Check sheet for the modelled part. Datum: model origin and axes. Units: mm. Face numbers are marked on the shaded views. A direction names the side the tool comes from. Coordinates: 2 decimals unless noted, no trailing zeros. Loops run counter-clockwise (first coordinate to the right, second up) from the corner with the lowest first, then second, coordinate; pieces in that order, holes last. Notation, with made-up numbers: (-26, 33) -> (-9, 33) arc R15 cw to (-9, 61) -> close; hole circle Ø10 at (19, 20.25). An arc over 180 degrees is marked (long way). Use CSV: the item, a comma, the result in double quotes. Start each with the question number.
1. Sectioned sample at D-D, the plane z = -16. Count the separate pieces of the cut face and the enclosed holes in it, and give its area (3 significant figures).
2. Sectioned sample at C-C, the plane y = -31. Record the cut outline in (x, z), and give its area (3 significant figures).
3. Thickness scan on L1, parallel to X at y = -71.1, z = -20; L2, parallel to X at y = -7.5, z = 33; L3, parallel to Y at x = -12.5, z = -45. Record the ranges inside material, lowest first.
4. Release check for a two-part mould opening along X. For the marked faces 3, 4 and 5 record: pulls with the +X half, pulls with the -X half, needs draft (parallel to the pull), parting line crosses it, or undercut.
5. Sectioned sample at A-A, the plane y = -4.5. Record the cut outline in (x, z), and give its area (3 significant figures).
6. Sectioned sample at B-B, the plane y = -54. Record the cut outline in (x, z).
7. Gauge pin test, flat ends, axial feed: pin 1 (1.8 mm diameter, centred on x = 25.81, z = -25.81, fed in from -Y); pin 2 (5 mm diameter, centred on x = 25.81, z = 25.81, fed in from +Y); pin 3 (8 mm diameter, centred on x = 10, z = 4.5, fed in from +Y). Record the tip position at first contact, or that the pin passes through.
8. Set-up check for the marked faces 1 and 2: record each of +Z, -Z, +X, -X, +Y, -Y from which the full face is reachable in a straight line by a thin tool's end or side.
```python
from build123d import *

# Parameters (mm, degrees)
SKETCH_1_W           = 90
SKETCH_1_H           = 80
SKETCH_1_R           = 30
EXTRUDE_1_DEPTH      = 4
SKETCH_2_R           = 1.5
CUT_EXTRUDE_1_DEPTH  = 4
SKETCH_3_W           = 80
SKETCH_3_H           = 80
EXTRUDE_2_DEPTH      = 4
SKETCH_4_W           = 80
SKETCH_4_H           = 80
EXTRUDE_3_DEPTH      = 4
SKETCH_5_R           = 1.5
CUT_EXTRUDE_2_DEPTH  = 4
SKETCH_6_R           = 20.5
CUT_EXTRUDE_3_DEPTH  = 4
SKETCH_8_W           = 98
SKETCH_8_H           = 80
EXTRUDE_4_DEPTH      = 4
SKETCH_9_R           = 8
CUT_EXTRUDE_5_DEPTH  = 4
SKETCH_10_R          = 2.75
CUT_EXTRUDE_6_DEPTH  = 2
SKETCH_11_W          = 106.087882822
SKETCH_11_H          = 86.695474134
CUT_EXTRUDE_7_DEPTH  = 2
SKETCH_12_W          = 90
SKETCH_12_H          = 80
EXTRUDE_5_DEPTH      = 2
SKETCH_13_W          = 115.80209227
SKETCH_13_H          = 95.07614962
CUT_EXTRUDE_8_DEPTH  = 0.5
SKETCH_14_R          = 12.5
CUT_EXTRUDE_9_DEPTH  = 4
FILLET_1_R           = 2
CUT_EXTRUDE_10_REACH = 131.151
SKETCH_15_R          = 10
SKETCH_16_W          = 90
SKETCH_16_H          = 70
EXTRUDE_6_DEPTH      = 10
SKETCH_17_W          = 90
SKETCH_17_H          = 70
EXTRUDE_7_DEPTH      = 10
SKETCH_19_R          = 2
CUT_EXTRUDE_12_DEPTH = 105.43778052
SKETCH_20_R          = 8
SKETCH_20_R_2        = 7.5
EXTRUDE_8_DEPTH      = 4


with BuildPart() as part:
    # 草图1 → 凸台-拉伸1 (new body)
    with BuildSketch(Plane(origin=(0, 0, 0), x_dir=(1, 0, 0), z_dir=(0, 1, 0))):
        Rectangle(SKETCH_1_W, SKETCH_1_H)
        with Locations(Location((0, 0, 0), (0, 0, 270))):
            Circle(SKETCH_1_R, mode=Mode.SUBTRACT)
    extrude(amount=EXTRUDE_1_DEPTH)

    # 草图2 → 切除-拉伸1 (cut)
    with BuildSketch(Plane(origin=(0, 4, 0), x_dir=(1, 0, 0), z_dir=(0, 1, 0))):
        with Locations(Location((0, 36.5, 0), (0, 0, 270))):
            Circle(SKETCH_2_R)
        with Locations(Location((25.809397513, 25.809397513, 0), (0, 0, 270))):
            Circle(SKETCH_2_R)
        with Locations(Location((36.5, 0, 0), (0, 0, 270))):
            Circle(SKETCH_2_R)
        with Locations(Location((25.809397513, -25.809397513, 0), (0, 0, 270))):
            Circle(SKETCH_2_R)
        with Locations(Location((0, -36.5, 0), (0, 0, 270))):
            Circle(SKETCH_2_R)
        with Locations(Location((-25.809397513, -25.809397513, 0), (0, 0, 270))):
            Circle(SKETCH_2_R)
        with Locations(Location((-36.5, 0, 0), (0, 0, 270))):
            Circle(SKETCH_2_R)
        with Locations(Location((-25.809397513, 25.809397513, 0), (0, 0, 270))):
            Circle(SKETCH_2_R)
    extrude(amount=-CUT_EXTRUDE_1_DEPTH, mode=Mode.SUBTRACT)

    # 草图3 → 凸台-拉伸2 (add)
    with BuildSketch(Plane(origin=(45, 0, 0), x_dir=(0, 0, -1), z_dir=(1, 0, 0))):
        with Locations((0, -36)):
            Rectangle(SKETCH_3_W, SKETCH_3_H)
    extrude(amount=EXTRUDE_2_DEPTH)

    # 草图4 → 凸台-拉伸3 (add)
    with BuildSketch(Plane.ZY.offset(45)):
        with Locations((0, -36)):
            Rectangle(SKETCH_4_W, SKETCH_4_H)
    extrude(amount=EXTRUDE_3_DEPTH)

    # 草图5 → 切除-拉伸2 (cut)
    with BuildSketch(Plane(origin=(49, 0, 0), x_dir=(0, 0, -1), z_dir=(1, 0, 0))):
        with Locations((-24, -36)):
            Circle(SKETCH_5_R)
        with Locations((-12, -15.215390309)):
            Circle(SKETCH_5_R)
        with Locations((12, -15.215390309)):
            Circle(SKETCH_5_R)
        with Locations((24, -36)):
            Circle(SKETCH_5_R)
        with Locations((12, -56.784609691)):
            Circle(SKETCH_5_R)
        with Locations((-12, -56.784609691)):
            Circle(SKETCH_5_R)
    extrude(amount=-CUT_EXTRUDE_2_DEPTH, mode=Mode.SUBTRACT)

    # 草图6 → 切除-拉伸3 (cut)
    with BuildSketch(Plane(origin=(49, 0, 0), x_dir=(0, 0, -1), z_dir=(1, 0, 0))):
        with Locations((0, -36)):
            Circle(SKETCH_6_R)
    extrude(amount=-CUT_EXTRUDE_3_DEPTH, mode=Mode.SUBTRACT)

    # 草图8 → 凸台-拉伸4 (add)
    with BuildSketch(Plane.XZ.offset(76)):
        Rectangle(SKETCH_8_W, SKETCH_8_H)
    extrude(amount=-EXTRUDE_4_DEPTH)

    # 草图9 → 切除-拉伸5 (cut)
    with BuildSketch(Plane.ZY.offset(49)):
        with Locations((0, -36)):
            Circle(SKETCH_9_R)
    extrude(amount=-CUT_EXTRUDE_5_DEPTH, mode=Mode.SUBTRACT)

    # 草图10 → 切除-拉伸6 (cut)
    with BuildSketch(Plane(origin=(0, 4, 0), x_dir=(1, 0, 0), z_dir=(0, 1, 0))):
        with Locations(Location((-25.809397513, 25.809397513, 0), (0, 0, 270))):
            Circle(SKETCH_10_R)
        with Locations(Location((0, 36.5, 0), (0, 0, 270))):
            Circle(SKETCH_10_R)
        with Locations(Location((25.809397513, 25.809397513, 0), (0, 0, 270))):
            Circle(SKETCH_10_R)
        with Locations(Location((36.5, 0, 0), (0, 0, 270))):
            Circle(SKETCH_10_R)
        with Locations(Location((25.809397513, -25.809397513, 0), (0, 0, 270))):
            Circle(SKETCH_10_R)
        with Locations(Location((0, -36.5, 0), (0, 0, 270))):
            Circle(SKETCH_10_R)
        with Locations(Location((-25.809397513, -25.809397513, 0), (0, 0, 270))):
            Circle(SKETCH_10_R)
        with Locations(Location((-36.5, 0, 0), (0, 0, 270))):
            Circle(SKETCH_10_R)
    extrude(amount=-CUT_EXTRUDE_6_DEPTH, mode=Mode.SUBTRACT)

    # 草图11 → 切除-拉伸7 (cut)
    with BuildSketch(Plane.XZ.offset(76)):
        with Locations((0.826302958, 0.912583938)):
            Rectangle(SKETCH_11_W, SKETCH_11_H)
    extrude(amount=-CUT_EXTRUDE_7_DEPTH, mode=Mode.SUBTRACT)

    # 草图12 → 凸台-拉伸5 (add)
    with BuildSketch(Plane(origin=(0, -72, 0), x_dir=(1, 0, 0), z_dir=(0, 1, 0))):
        Rectangle(SKETCH_12_W, SKETCH_12_H)
    extrude(amount=EXTRUDE_5_DEPTH)

    # 草图13 → 切除-拉伸8 (cut)
    with BuildSketch(Plane(origin=(0, 4, 0), x_dir=(1, 0, 0), z_dir=(0, 1, 0))):
        with Locations((-2.14666103, 3.125340558)):
            Rectangle(SKETCH_13_W, SKETCH_13_H)
    extrude(amount=-CUT_EXTRUDE_8_DEPTH, mode=Mode.SUBTRACT)

    # 草图14 → 切除-拉伸9 (cut)
    with BuildSketch(Plane.XZ.offset(74)):
        with Locations(Location((-29, 20, 0), (0, 0, 270))):
            Circle(SKETCH_14_R)
        with Locations(Location((29, 20, 0), (0, 0, 270))):
            Circle(SKETCH_14_R)
        with Locations(Location((0, 0, 0), (0, 0, 270))):
            Circle(SKETCH_14_R)
        with Locations(Location((-29, -20, 0), (0, 0, 270))):
            Circle(SKETCH_14_R)
        with Locations(Location((29, -20, 0), (0, 0, 270))):
            Circle(SKETCH_14_R)
    extrude(amount=-CUT_EXTRUDE_9_DEPTH, mode=Mode.SUBTRACT)

    # 圆角1
    fillet_1_edges = [part.edges().sort_by_distance(p)[0] for p in [
        (-49, -74, 0),
        (49, -74, 0),
        (49, 3.5, 0),
        (-49, 3.5, 0),
    ]]
    fillet(fillet_1_edges, radius=FILLET_1_R)

    # 草图15 → 切除-拉伸10 (cut, up to next)
    with BuildSketch(Plane.ZY.offset(49), mode=Mode.PRIVATE) as cut_extrude_10_sk1:
        with Locations((-20, -16.5)):
            Circle(SKETCH_15_R)
    cut_extrude_10_tool1 = extrude(cut_extrude_10_sk1.sketch, amount=-CUT_EXTRUDE_10_REACH, mode=Mode.PRIVATE) & part.part
    # 草图15 → 切除-拉伸10 (cut, up to next)
    with BuildSketch(Plane.ZY.offset(49), mode=Mode.PRIVATE) as cut_extrude_10_sk2:
        with Locations((20, -16.5)):
            Circle(SKETCH_15_R)
    cut_extrude_10_tool2 = extrude(cut_extrude_10_sk2.sketch, amount=-CUT_EXTRUDE_10_REACH, mode=Mode.PRIVATE) & part.part
    # 草图15 → 切除-拉伸10 (cut, up to next)
    with BuildSketch(Plane.ZY.offset(49), mode=Mode.PRIVATE) as cut_extrude_10_sk3:
        with Locations((20, -54)):
            Circle(SKETCH_15_R)
    cut_extrude_10_tool3 = extrude(cut_extrude_10_sk3.sketch, amount=-CUT_EXTRUDE_10_REACH, mode=Mode.PRIVATE) & part.part
    # 草图15 → 切除-拉伸10 (cut, up to next)
    with BuildSketch(Plane.ZY.offset(49), mode=Mode.PRIVATE) as cut_extrude_10_sk4:
        with Locations((-20, -54)):
            Circle(SKETCH_15_R)
    cut_extrude_10_tool4 = extrude(cut_extrude_10_sk4.sketch, amount=-CUT_EXTRUDE_10_REACH, mode=Mode.PRIVATE) & part.part
    add(cut_extrude_10_tool1.solids().sort_by_distance((-49, -16.5, -20))[0], mode=Mode.SUBTRACT)
    add(cut_extrude_10_tool2.solids().sort_by_distance((-49, -16.5, 20))[0], mode=Mode.SUBTRACT)
    add(cut_extrude_10_tool3.solids().sort_by_distance((-49, -54, 20))[0], mode=Mode.SUBTRACT)
    add(cut_extrude_10_tool4.solids().sort_by_distance((-49, -54, -20))[0], mode=Mode.SUBTRACT)

    # 草图16 → 凸台-拉伸6 (add)
    with BuildSketch(Plane(origin=(0, 0, -40), x_dir=(-1, 0, 0), z_dir=(0, 0, -1))):
        with BuildLine():
            Line((-47, -74), (47, -74))
            ThreePointArc((47, -74), (48.414213562, -73.414213562), (49, -72))
            Line((49, -72), (49, 1.5))
            ThreePointArc((49, 1.5), (48.414213562, 2.914213562), (47, 3.5))
            Line((47, 3.5), (-47, 3.5))
            ThreePointArc((-47, 3.5), (-48.414213562, 2.914213562), (-49, 1.5))
            Line((-49, 1.5), (-49, -72))
            ThreePointArc((-49, -72), (-48.414213562, -73.414213562), (-47, -74))
        make_face()
        with Locations((0, -35)):
            Rectangle(SKETCH_16_W, SKETCH_16_H, mode=Mode.SUBTRACT)
    extrude(amount=EXTRUDE_6_DEPTH)

    # 草图17 → 凸台-拉伸7 (add)
    with BuildSketch(Plane.XY.offset(40)):
        with BuildLine():
            Line((-49, 1.5), (-49, -72))
            ThreePointArc((-49, -72), (-48.414213562, -73.414213562), (-47, -74))
            Line((-47, -74), (47, -74))
            ThreePointArc((47, -74), (48.414213562, -73.414213562), (49, -72))
            Line((49, -72), (49, 1.5))
            ThreePointArc((49, 1.5), (48.414213562, 2.914213562), (47, 3.5))
            Line((47, 3.5), (-47, 3.5))
            ThreePointArc((-47, 3.5), (-48.414213562, 2.914213562), (-49, 1.5))
        make_face()
        with Locations((0, -35)):
            Rectangle(SKETCH_17_W, SKETCH_17_H, mode=Mode.SUBTRACT)
    extrude(amount=EXTRUDE_7_DEPTH)

    # 草图19 → 切除-拉伸12 (cut, through all)
    with BuildSketch(Plane.XZ.offset(74)):
        with Locations(Location((37, -38, 0), (0, 0, 90))):
            Circle(SKETCH_19_R)
        with Locations(Location((-37, 38, 0), (0, 0, 270))):
            Circle(SKETCH_19_R)
        with Locations(Location((37, 38, 0), (0, 0, 270))):
            Circle(SKETCH_19_R)
        with Locations(Location((-37, -38, 0), (0, 0, 90))):
            Circle(SKETCH_19_R)
    extrude(amount=-CUT_EXTRUDE_12_DEPTH, mode=Mode.SUBTRACT)

    # 草图20 → 凸台-拉伸8 (add)
    with BuildSketch(Plane.ZY.offset(49)):
        with Locations((0, -36)):
            Circle(SKETCH_20_R)
        with Locations((0, -36)):
            Circle(SKETCH_20_R_2, mode=Mode.SUBTRACT)
    extrude(amount=-EXTRUDE_8_DEPTH)


solid = part.part
```
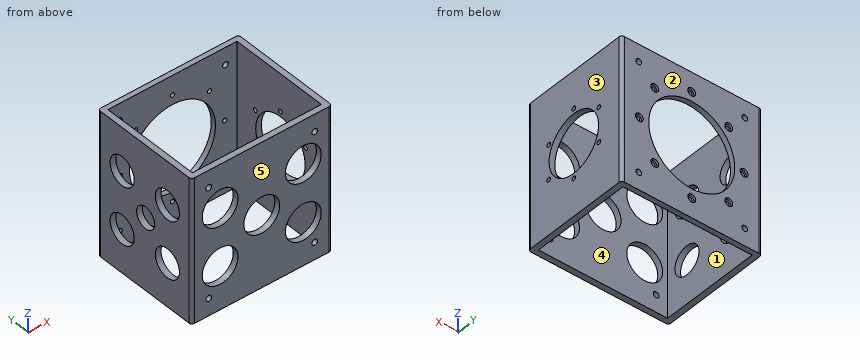
Completed:
1,separate pieces,"6"
1,enclosed holes,"0"
1,area,"675 mm²"
2,outline,"(-49, -50) -> (-45, -50) -> (-45, -5.59) -> (-49, -5.59) -> close; (-49, 5.59) -> (-45, 5.59) -> (-45, 50) -> (-49, 50) -> close; (45, -50) -> (49, -50) -> (49, -19.88) -> (45, -19.88) -> close; (45, 19.88) -> (49, 19.88) -> (49, 50) -> (45, 50) -> close"
2,area,"596 mm²"
3,L1,"-49 to -41.5, -16.5 to 16.5, 41.5 to 49"
3,L2,"-49 to -45, 45 to 49"
3,L3,"-74 to -70, 0 to 3.5"
4,face 3,"pulls with the +X half"
4,face 4,"undercut"
4,face 5,"needs draft"
5,outline,"(-49, -50) -> (-45, -50) -> (-45, 50) -> (-49, 50) -> close; (45, -50) -> (49, -50) -> (49, 50) -> (45, 50) -> close"
5,area,"800 mm²"
6,outline,"(-49, -50) -> (-45, -50) -> (-45, -30) -> (-49, -30) -> close; (-49, -10) -> (-45, -10) -> (-45, 10) -> (-49, 10) -> close; (-49, 30) -> (-45, 30) -> (-45, 50) -> (-49, 50) -> close; (45, -50) -> (49, -50) -> (49, -9.81) -> (45, -9.81) -> close; (45, 9.81) -> (49, 9.81) -> (49, 50) -> (45, 50) -> close"
7,pin 1,"through"
7,pin 2,"y = 2"
7,pin 3,"y = -70"
8,face 1,"+Z, -Z"
8,face 2,"+Z, -Z, +X, -X, +Y"
